Here's the drawing with two shaded views (mm, measured from the low corner). I have some questions. Coordinates: 2 decimals unless noted, no trailing zeros. Write each loop counter-clockwise with the first axis right and the second up, starting at its lowest first coordinate (ties: lowest second). Pieces come first, ordered by that corner, then holes. Notation, with made-up numbers: (-39, -1) -> (-21, -1) arc R27 cw to (-21, 28) -> close; hole circle Ø10 at (6, -5.75). An arc over 180 degrees is marked (long way). Answer in a Markdown table with one row per item. Add a question column.
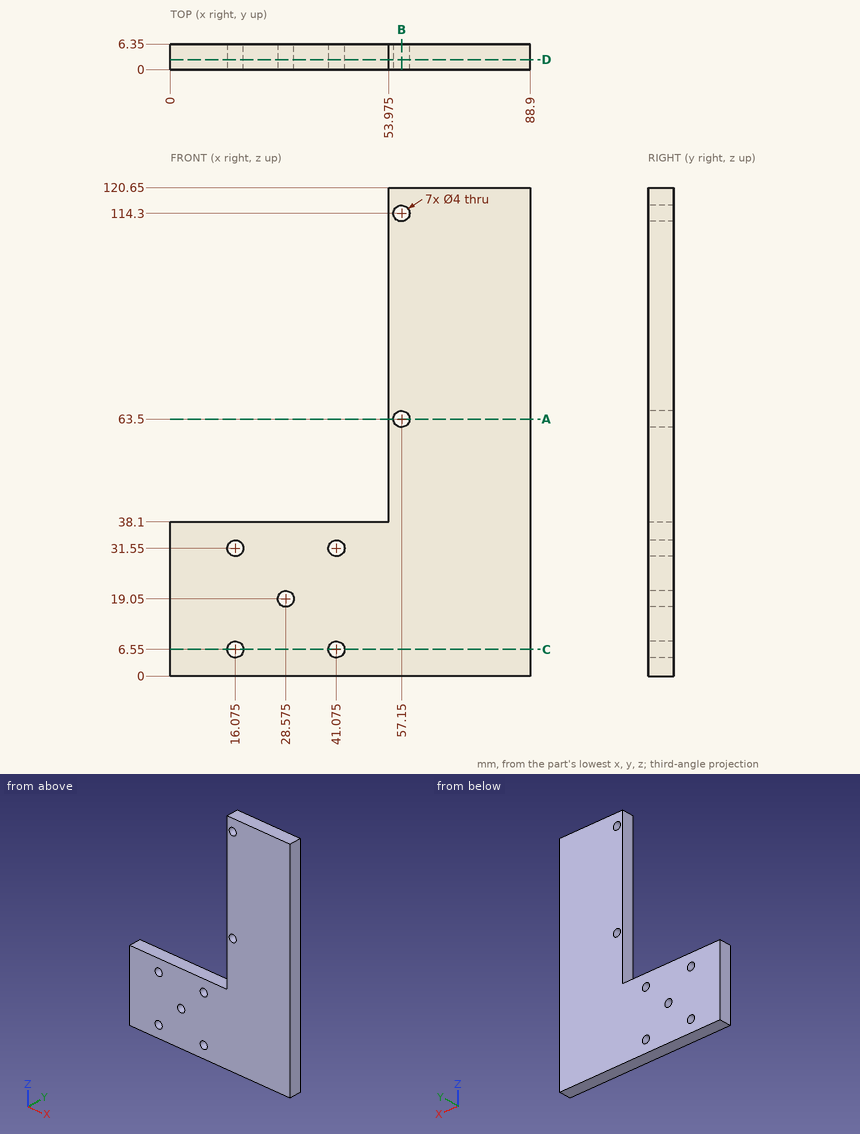
Q1. Imagine slicing it at D-D on y = 2.5. Please give me the cut outline in (x, z) (3 decimals), plus the area to 3 significant figures.
Q2. Imagine slicing it at C-C on z = 6.55. Please give me the cut outline in (x, y) (3 decimals).
Q3. Imagine slicing it at B-B on x = 57.15. Please give me the cut outline in (y, z), plus the area to 3 significant figures.
Q4. Imagine slicing it at A-A on z = 63.5. Please give me the cut outline in (x, y) (3 decimals).
Q5. I need wall thicknesses on line 1 (Z direction, x = 57, y = 0.5); line 2 (X direction, y = 5.5, z = 30); line 3 (Z direction, x = 45, y = 3). Which ranges of each line are inside material? Lowest first, please. Write a range as [from, to].
Result sheet:
| question | item | result |
|---|---|---|
| 1 | outline | (0, 0) -> (88.9, 0) -> (88.9, 120.65) -> (53.975, 120.65) -> (53.975, 38.1) -> (0, 38.1) -> close; hole circle Ø4 at (16.075, 6.55); hole circle Ø4 at (16.075, 31.55); hole circle Ø4 at (28.575, 19.05); hole circle Ø4 at (41.075, 6.55); hole circle Ø4 at (41.075, 31.55); hole circle Ø4 at (57.15, 63.5); hole circle Ø4 at (57.15, 114.3) |
| 1 | area | 6,180 mm^2 |
| 2 | outline | (0, 0) -> (14.075, 0) -> (14.075, 6.35) -> (0, 6.35) -> close; (18.075, 0) -> (39.075, 0) -> (39.075, 6.35) -> (18.075, 6.35) -> close; (43.075, 0) -> (88.9, 0) -> (88.9, 6.35) -> (43.075, 6.35) -> close |
| 3 | outline | (0, 0) -> (6.35, 0) -> (6.35, 61.5) -> (0, 61.5) -> close; (0, 65.5) -> (6.35, 65.5) -> (6.35, 112.3) -> (0, 112.3) -> close; (0, 116.3) -> (6.35, 116.3) -> (6.35, 120.65) -> (0, 120.65) -> close |
| 3 | area | 715 mm^2 |
| 4 | outline | (53.975, 0) -> (55.15, 0) -> (55.15, 6.35) -> (53.975, 6.35) -> close; (59.15, 0) -> (88.9, 0) -> (88.9, 6.35) -> (59.15, 6.35) -> close |
| 5 | line 1 | z = [0, 61.51], [65.49, 112.31], [116.29, 120.65] |
| 5 | line 2 | x = [0, 14.81], [17.34, 39.81], [42.34, 88.9] |
| 5 | line 3 | z = [0, 38.1] |
